Could you check a few things on this model? Use its own coordinates, in mm. Face numbers are marked on the shaded views. Give positions to 0.01 mm unless a question says otherwise; leave off trailing zeros. Write each loop counter-clockwise with the first axis right and the second up, starting at its lowest first coordinate (ties: lowest second). Pieces come first, ordered by that corner, then holes. Notation, with made-up numbers: M 20.25,-31 L 65.25,-31 A23 cw 65.25,-9 Z; hole C 37.5,75 d3. An arc over 180 degrees is marked long. Use one line per item in the form item = value.
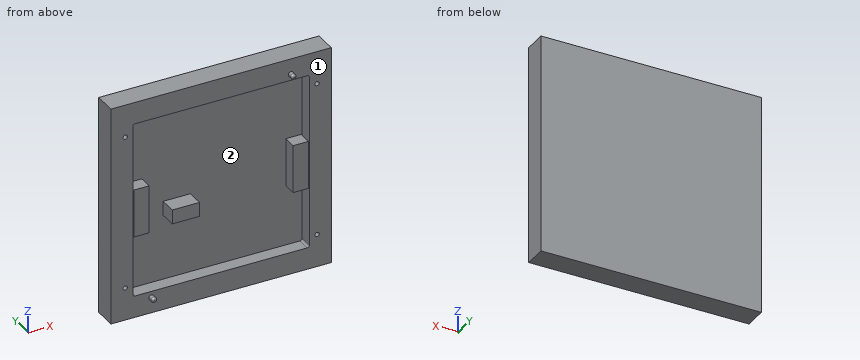
from build123d import *

# Parameters (mm, degrees)
SKETCH1_W           = 127.9906
SKETCH1_H           = 127.8382
BOSS_EXTRUDE1_DEPTH = 13.1826
SKETCH2_W           = 102.5906
SKETCH2_H           = 102.4382
CUT_EXTRUDE1_DEPTH  = 7.874
SKETCH3_R           = 1.27
CUT_EXTRUDE2_DEPTH  = 7.874
SKETCH4_W           = 15.7988
SKETCH4_H           = 8.2804
BOSS_EXTRUDE2_DEPTH = 9.8298
SKETCH5_W           = 8.89
SKETCH5_H           = 27.94
BOSS_EXTRUDE3_DEPTH = 7.874
SKETCH6_R           = 1.5113
BOSS_EXTRUDE4_DEPTH = 3.683
FILLET3_R           = 1.27
FILLET4_R           = 1.27
FILLET5_R           = 1.27
FILLET6_R           = 1.27
FILLET8_R           = 1.27
FILLET9_R           = 1.27


with BuildPart() as part:
    # Sketch1 → Boss-Extrude1 (new body)
    with BuildSketch(Plane(origin=(0, 0, 0), x_dir=(1, 0, 0), z_dir=(0, 1, 0))):
        with Locations((63.9953, 63.9191)):
            Rectangle(SKETCH1_W, SKETCH1_H)
    extrude(amount=BOSS_EXTRUDE1_DEPTH)

    # Sketch2 → Cut-Extrude1 (cut)
    with BuildSketch(Plane.XZ):
        with Locations((63.9953, -63.9191)):
            Rectangle(SKETCH2_W, SKETCH2_H)
    extrude(amount=-CUT_EXTRUDE1_DEPTH, mode=Mode.SUBTRACT)

    # Sketch3 → Cut-Extrude2 (cut)
    with BuildSketch(Plane.XZ):
        with Locations((8.255, -108.7882)):
            Circle(SKETCH3_R)
        with Locations((8.255, -19.05)):
            Circle(SKETCH3_R)
        with Locations((119.7356, -108.7882)):
            Circle(SKETCH3_R)
        with Locations((119.7356, -19.05)):
            Circle(SKETCH3_R)
    extrude(amount=-CUT_EXTRUDE2_DEPTH, mode=Mode.SUBTRACT)

    # Sketch4 → Boss-Extrude2 (add)
    with BuildSketch(Plane(origin=(0, 7.874, 0), x_dir=(-1, 0, 0), z_dir=(0, -1, 0))):
        with Locations((-42.4688, 72.9996)):
            Rectangle(SKETCH4_W, SKETCH4_H)
    extrude(amount=BOSS_EXTRUDE2_DEPTH)

    # Sketch5 → Boss-Extrude3 (add)
    with BuildSketch(Plane(origin=(0, 7.874, 0), x_dir=(-1, 0, 0), z_dir=(0, -1, 0))):
        with Locations((-17.7292, 65.9384)):
            Rectangle(SKETCH5_W, SKETCH5_H)
        with Locations((-110.2614, 65.9384)):
            Rectangle(SKETCH5_W, SKETCH5_H)
    extrude(amount=BOSS_EXTRUDE3_DEPTH)

    # Sketch6 → Boss-Extrude4 (add)
    with BuildSketch(Plane(origin=(0, 0, 0), x_dir=(-1, 0, 0), z_dir=(0, -1, 0))):
        with Locations((-23.4823, 118.7323)):
            Circle(SKETCH6_R)
        with Locations((-104.5083, 9.1059)):
            Circle(SKETCH6_R)
    extrude(amount=BOSS_EXTRUDE4_DEPTH)

    # Fillet3
    fillet3_edges = [part.edges().sort_by_distance(p)[0] for p in [
        (12.7, 3.937, -115.1382),
    ]]
    fillet(fillet3_edges, radius=FILLET3_R)

    # Fillet4
    fillet4_edges = [part.edges().sort_by_distance(p)[0] for p in [
        (12.7, 3.937, -12.7),
    ]]
    fillet(fillet4_edges, radius=FILLET4_R)

    # Fillet5
    fillet5_edges = [part.edges().sort_by_distance(p)[0] for p in [
        (115.2906, 3.937, -12.7),
    ]]
    fillet(fillet5_edges, radius=FILLET5_R)

    # Fillet6
    fillet6_edges = [part.edges().sort_by_distance(p)[0] for p in [
        (115.2906, 3.937, -115.1382),
    ]]
    fillet(fillet6_edges, radius=FILLET6_R)

    # Fillet8
    fillet8_edges = [part.edges().sort_by_distance(p)[0] for p in [
        (24.9936, -3.683, -118.7323),
    ]]
    fillet(fillet8_edges, radius=FILLET8_R)

    # Fillet9
    fillet9_edges = [part.edges().sort_by_distance(p)[0] for p in [
        (106.0196, -3.683, -9.1059),
    ]]
    fillet(fillet9_edges, radius=FILLET9_R)


solid = part.part
1) I want a section at D-D, the plane x = 11. Please give me the cut outline in (y, z).
Checked values:
outline = M 0,-127.84 L 13.18,-127.84 L 13.18,0 L 0,0 Z
2) I want a section at A-A, the plane y = 4.5. Count the separate pieces of the cut face and the enclosed holes in it, plus the area to 3 significant figures.
Checked values:
separate_pieces = 4
enclosed_holes = 5
area = 6,460 mm2
3) I want a section at C-C, the plane z = -93.5. Please give me the cut outline in (x, y), plus the area to 3 significant figures.
Checked values:
outline = M 0,0 L 12.7,0 L 12.7,7.87 L 115.29,7.87 L 115.29,0 L 127.99,0 L 127.99,13.18 L 0,13.18 Z
area = 879 mm2
4) Thinking about a two-plate mould opening in X: for the marked faces 1 and 2, which applies, released by +X, released by -X, zero draft, split by the parting line, or undercut?
Checked values:
face_1 = zero draft
face_2 = undercut
5) I want a section at B-B, the plane x = 62. Please give me the cut outline in (y, z).
Checked values:
outline = M 0,-127.84 L 13.18,-127.84 L 13.18,0 L 0,0 L 0,-12.7 L 7.87,-12.7 L 7.87,-115.14 L 0,-115.14 Z
6) For pin 1 Ø4 at (x, z) = (8.255, -19.05) entering from -Y; pin 2 Ø0.8 at (x, z) = (120, -108.5) entering from -Y, each with a flat end and sliding along its axis, tell me the tip position at first contact or that it passes through.
Checked values:
pin_1 = 0
pin_2 = 7.87
7) If I drill on L1, parallel to Z at x = 39, y = 6.5; L2, parallel to X at y = 5, z = -65.5; L3, parallel to X at y = 2.75, z = -77, over which ranges is the centre line in solid material (lowest first)?
Checked values:
L1 = -127.84 to -115.14, -77.14 to -68.86, -12.7 to 0
L2 = 0 to 12.7, 13.28 to 22.17, 105.82 to 114.71, 115.29 to 127.99
L3 = 0 to 12.7, 13.28 to 22.17, 34.57 to 50.37, 105.82 to 114.71, 115.29 to 127.99
